Read the model definition and answer for the solid it produces. Units are mm, in the model's axes. Face numbers are marked on the shaded views. Coordinates: 2 decimals unless noted, no trailing zeros. Order: outer loops, then holes, each group sorted by start corner. A loop starts at its lowest first (then second) coordinate and runs counter-clockwise, first axis right, second up. Notation, with made-up numbers: (74, 11) -> (105, 11) arc R37 cw to (105, 48) -> close; hole circle Ø11 at (66, 54). An arc over 180 degrees is marked (long way). Answer as a JSON object with one key per item and string values. Group by question number.
1) Section A-A on x = 0 is taken. Determine the outline of the cut face in (y, z).
2) Given pin 1 (2.5 mm diameter, centred on x = 0, z = 0, fed in from -Y); pin 2 (6 mm diameter, centred on x = -4.5, y = 19, fed in from -Z); pin 3 (1.5 mm diameter, centred on x = 4, y = 22, fed in from +Z), each flat-ended and moving along its own axis, determine where each tip first touches the part or whether it passes through.
3) Section B-B on z = 0 is taken. Determine the outline of the cut face in (x, y), and give its area (3 significant figures).
4) Section C-C on y = 15.75 is taken. Determine the outline of the cut face in (x, z), and give its area (3 significant figures).
5) Consider L1, parallel to X at y = 16, z = 0; L2, parallel to X at y = 7.75, z = 0; L3, parallel to X at y = 19.5, z = 5. Determine where each line is inside the solid, lowest interval first.
6) Determine the mould class of the marked faces 1, 2, 3 and 4 for opening direction Z: released by +Z, released by -Z, zero draft, split by the parting line, or undercut.
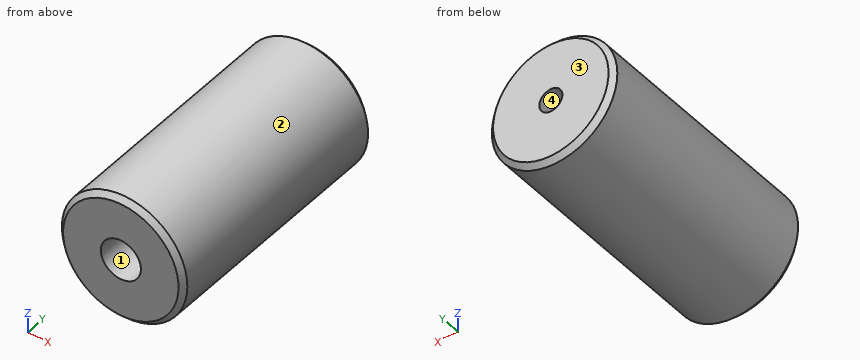
from build123d import *

# Parameters (mm, degrees)
SKETCH2_R           = 6.25
BOSS_EXTRUDE1_DEPTH = 9
SKETCH3_R           = 6.25
BOSS_EXTRUDE2_DEPTH = 7
SKETCH4_R           = 6.25
BOSS_EXTRUDE3_DEPTH = 9
SKETCH5_R           = 2
CUT_EXTRUDE1_DEPTH  = 12.5
SKETCH6_R           = 1.15
CUT_EXTRUDE2_DEPTH  = 12.5
CHAMFER2_SIZE       = 0.5


with BuildPart() as part:
    # Sketch2 → Boss-Extrude1 (new body)
    with BuildSketch(Plane(origin=(0, 0, 0), x_dir=(1, 0, 0), z_dir=(0, 1, 0))):
        with Locations(Location((0, 0, 0), (0, 0, 270))):
            Circle(SKETCH2_R)
    extrude(amount=BOSS_EXTRUDE1_DEPTH)

    # Sketch3 → Boss-Extrude2 (add)
    with BuildSketch(Plane(origin=(0, 9, 0), x_dir=(1, 0, 0), z_dir=(0, 1, 0))):
        with Locations(Location((0, 0, 0), (0, 0, 270))):
            Circle(SKETCH3_R)
    extrude(amount=BOSS_EXTRUDE2_DEPTH)

    # Sketch4 → Boss-Extrude3 (add)
    with BuildSketch(Plane(origin=(0, 16, 0), x_dir=(1, 0, 0), z_dir=(0, 1, 0))):
        with Locations(Location((0, 0, 0), (0, 0, 270))):
            Circle(SKETCH4_R)
    extrude(amount=BOSS_EXTRUDE3_DEPTH)

    # Sketch5 → Cut-Extrude1 (cut)
    with BuildSketch(Plane.XZ):
        with Locations(Location((0, 0, 0), (0, 0, 270))):
            Circle(SKETCH5_R)
    extrude(amount=-CUT_EXTRUDE1_DEPTH, mode=Mode.SUBTRACT)

    # Sketch6 → Cut-Extrude2 (cut)
    with BuildSketch(Plane(origin=(0, 25, 0), x_dir=(1, 0, 0), z_dir=(0, 1, 0))):
        with Locations(Location((0, 0, 0), (0, 0, 270))):
            Circle(SKETCH6_R)
    extrude(amount=-CUT_EXTRUDE2_DEPTH, mode=Mode.SUBTRACT)

    # Chamfer2
    chamfer2_edges = [part.edges().sort_by_distance(p)[0] for p in [
        (0, 25, -6.25),
        (0, 0, -6.25),
    ]]
    chamfer(chamfer2_edges, length=CHAMFER2_SIZE)


solid = part.part
Worked answers:
{
 "1": {"outline": "(0, -5.75) -> (0.5, -6.25) -> (24.5, -6.25) -> (25, -5.75) -> (25, -1.15) -> (12.5, -1.15) -> (12.5, -2) -> (0, -2) -> close; (0, 2) -> (12.5, 2) -> (12.5, 1.15) -> (25, 1.15) -> (25, 5.75) -> (24.5, 6.25) -> (0.5, 6.25) -> (0, 5.75) -> close"},
 "2": {"pin 1": "stops at y = 12.5", "pin 2": "stops at z = -6.07", "pin 3": "stops at z = 5.34"},
 "3": {"outline": "(-6.25, 0.5) -> (-5.75, 0) -> (-2, 0) -> (-2, 12.5) -> (-1.15, 12.5) -> (-1.15, 25) -> (-5.75, 25) -> (-6.25, 24.5) -> close; (1.15, 12.5) -> (2, 12.5) -> (2, 0) -> (5.75, 0) -> (6.25, 0.5) -> (6.25, 24.5) -> (5.75, 25) -> (1.15, 25) -> close", "area": "233 mm²"},
 "4": {"outline": "circle Ø12.5 at (0, 0); hole circle Ø2.3 at (0, 0)", "area": "119 mm²"},
 "5": {"L1": "x = -6.25 to -1.15, 1.15 to 6.25", "L2": "x = -6.25 to -2, 2 to 6.25", "L3": "x = -3.75 to 3.75"},
 "6": {"face 1": "undercut", "face 2": "split by the parting line", "face 3": "zero draft", "face 4": "undercut"}
}
